Source: CAD feature listing. Evaluate the final solid. Frame: model axes, mm. Face numbers are marked on the shaded views. A direction names the side the tool comes from. Give positions to 0.01 mm unless a question says otherwise; leave off trailing zeros. Write each loop counter-clockwise with the first axis right and the second up, starting at its lowest first coordinate (ties: lowest second). Pieces come first, ordered by that corner, then holes.
```python
from build123d import *

# Parameters (mm, degrees)
SKETCH2_R                = 7.9375
BOSS_EXTRUDE1_DEPTH      = 6.35
SKETCH3_R                = 7.0485
BOSS_EXTRUDE2_DEPTH      = 15.113
SKETCH4_W                = 5.588
SKETCH4_H                = 2.76225
CUT_EXTRUDE1_DEPTH       = 6.35
F_5_16_24_TAPPED_HOLE1_D = 6.9088


with BuildPart() as part:
    # Sketch2 → Boss-Extrude1 (new body)
    with BuildSketch(Plane(origin=(0, 0, 0), x_dir=(0, 0, -1), z_dir=(1, 0, 0))):
        Circle(SKETCH2_R)
    extrude(amount=-BOSS_EXTRUDE1_DEPTH)

    # Sketch3 → Boss-Extrude2 (add)
    with BuildSketch(Plane(origin=(0, 0, 0), x_dir=(0, 0, -1), z_dir=(1, 0, 0))):
        Circle(SKETCH3_R)
    extrude(amount=BOSS_EXTRUDE2_DEPTH)

    # Sketch4 → Cut-Extrude1 (cut, symmetric)
    with BuildSketch(Plane(origin=(0, 0, 0), x_dir=(1, 0, 0), z_dir=(0, 1, 0))):
        with Locations((-3.556, 6.556375)):
            Rectangle(SKETCH4_W, SKETCH4_H)
        with Locations((-3.556, -6.556375)):
            Rectangle(SKETCH4_W, SKETCH4_H)
    extrude(amount=CUT_EXTRUDE1_DEPTH, both=True, mode=Mode.SUBTRACT)

    # 5/16-24 Tapped Hole1 (through all)
    with Locations(Plane(origin=(-6.35, 0, 0), x_dir=(0, 0, -1), z_dir=(-1, 0, 0))):
        with Locations((0, 0)):
            Hole(F_5_16_24_TAPPED_HOLE1_D / 2)


solid = part.part
```
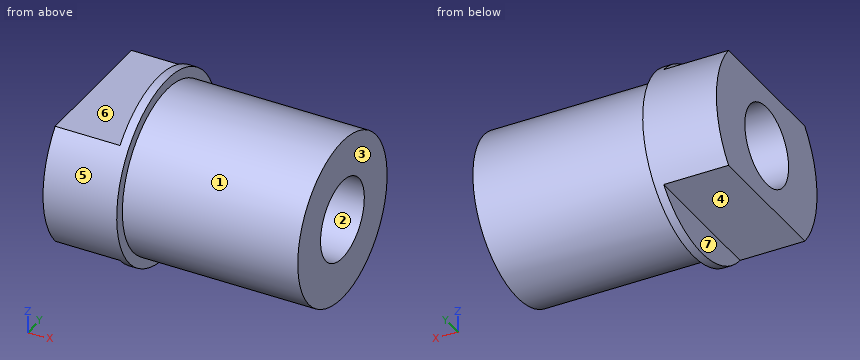
1. Line query: probe 1 along Y at (x, z) = (3, 0); probe 2 along X at (y, z) = (-0.75, 6.25); probe 3 along Z at (x, y) = (-1.25, 1.25). Output: solid intervals per line, ascending.
2. Section query A-A (z = 0). Return loops of the section in (x, y).
3. Section query B-B (y = 0). Return loops of the section in (x, z), plus the area to 3 significant figures.
4. Section query C-C (x = -3.25). Return loops of the section in (y, z) (1 decimal).
5. Access query for the marked faces 5, 6 and 7. Directions: +Z, -Z, +X, -X, +Y, -Y. A direction counts if a zero-diameter tool reaches every point of the face in a straight line with its end or side. Return the directions, or none.
6. Section query D-D (y = -4). Return loops of the section in (x, z).
7. Pin query (flat end, axial travel): P1, Ø0.8, axis at y = -1, z = -7, coming from the -X side; P2, Ø4.5, axis at x = -4.5, y = -1, coming from the +Z side; P3, Ø4, axis at x = 5.5, z = -4, coming from the +Y side; P4, Ø1, axis at y = 0, z = 2.5, coming from the -X side. Return the tip coordinate at first contact, or that it passes through.
8. Pull-direction query (Z, two-part tool) for the marked faces 1, 2, 3 and 4; classes: pulls with the +Z half, pulls with the -Z half, needs draft (parallel to the pull), parting line crosses it, or undercut.
The answers:
1. probe 1: y = -7.05 to -3.45, 3.45 to 7.05
1. probe 2: x = -0.76 to 15.11
1. probe 3: z = -5.18 to -3.22, 3.22 to 5.18
2. outline: (-6.35, -7.94) - (0, -7.94) - (0, -7.05) - (15.11, -7.05) - (15.11, -3.45) - (-6.35, -3.45) - close; (-6.35, 3.45) - (15.11, 3.45) - (15.11, 7.05) - (0, 7.05) - (0, 7.94) - (-6.35, 7.94) - close
3. outline: (-6.35, -5.18) - (-0.76, -5.18) - (-0.76, -7.94) - (0, -7.94) - (0, -7.05) - (15.11, -7.05) - (15.11, -3.45) - (-6.35, -3.45) - close; (-6.35, 3.45) - (15.11, 3.45) - (15.11, 7.05) - (0, 7.05) - (0, 7.94) - (-0.76, 7.94) - (-0.76, 5.18) - (-6.35, 5.18) - close
3. area: 135 mm2
4. outline: (-6, -5.2) - (6, -5.2) arc R7.9 ccw to (6, 5.2) - (-6, 5.2) arc R7.9 ccw to start; hole circle Ø6.9 at (0, 0)
5. face 5: +X, -X
5. face 6: +Z, -X, +Y, -Y
5. face 7: -Z, -X, +Y, -Y
6. outline: (-6.35, -5.18) - (-0.76, -5.18) - (-0.76, -6.86) - (0, -6.86) - (0, -5.8) - (15.11, -5.8) - (15.11, 5.8) - (0, 5.8) - (0, 6.86) - (-0.76, 6.86) - (-0.76, 5.18) - (-6.35, 5.18) - close
7. P1: stops at x = -0.76
7. P2: stops at z = 5.18
7. P3: stops at y = 6.76
7. P4: passes through
8. face 1: parting line crosses it
8. face 2: undercut
8. face 3: needs draft
8. face 4: pulls with the -Z half
